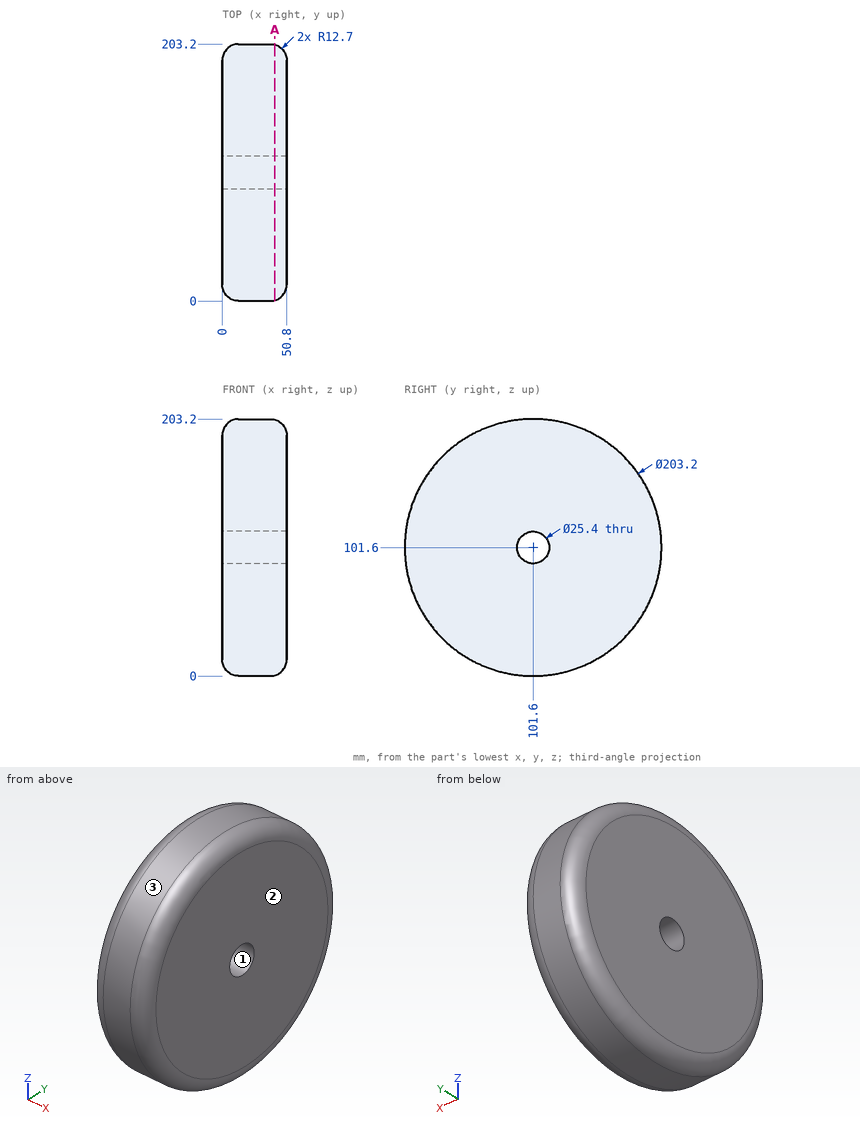
Part print with two shaded views. Sizes in mm from the minimum x, y, z corner. Give positions to 0.01 mm unless a question says otherwise; leave off trailing zeros. Order: outer loops, then holes, each group sorted by start corner. A loop starts at its lowest first (then second) coordinate and runs counter-clockwise, first axis right, second up. Notation, with made-up numbers: M 58,26 L 74,26 A26 ccw 74,47 Z; hole C 59,-25.5 d8. An arc over 180 degrees is marked long. Put each result on its own line as item: value.
Item 1: Wall check: probe 1 along Z at (x, y) = (30.5, 101.6); probe 2 along Y at (x, z) = (15, 101); probe 3 along Y at (x, z) = (36.5, 97.5). Give the ranges that are in metal, low to high.
Results are:
probe 1: 0 to 88.9, 114.3 to 203.2
probe 2: 0 to 88.91, 114.29 to 203.2
probe 3: 0.08 to 89.58, 113.62 to 203.12
Item 2: Drop flat-ended pins along their axis: pin 1 Ø10 at (x, z) = (6.5, 162) entering from -Y; pin 2 Ø10 at (x, y) = (7, 53.5) entering from -Z; pin 3 Ø10 at (x, z) = (21, 35) entering from -Y. Give the stop position or say it passes through.
Results are:
pin 1: y = 17.53
pin 2: z = 10.37
pin 3: y = 20.8
Item 3: Pull direction Z, two halves, no side cores. Call the marked faces 1, 2 and 3: +Z half, -Z half, draft (parallel to the pull), parting line (faces both ways), or undercut.
Results are:
face 1: undercut
face 2: draft
face 3: parting line
Item 4: Cut at A-A on x = 41.5. Write the cut outline in (y, z), then the cut area to 3 significant figures.
Results are:
outline: C 101.6,101.6 d202.27; hole C 101.6,101.6 d25.4
area: 31,600 mm2
